Build history of the part. All positions in model axes, mm. A direction names the side the tool comes from. Coordinates: 2 decimals unless noted, no trailing zeros. Loops run counter-clockwise (first coordinate to the right, second up) from the corner with the lowest first, then second, coordinate; pieces in that order, holes last.
Item 1: Mould opens along X. For faces 3 (the face through (21, 2.54, -19)), 4 (the face through (0, 6.35, -19)), 5 (the face through (19.32, 1.25, -6.26)) say: released by +X, released by -X, zero draft, split by the parting line, or undercut.
Item 2: Cut at B-B (x = 25). List the corners of the cut face in (y, z), and give its area (3 significant figures).
Item 3: Flat gauge pins, fed straight in: pin 1 (2 mm diameter, centred on x = 20.5, y = 2.5, fed in from -Z); pin 2 (1.5 mm diameter, centred on y = 7.5, z = -30, fed in from +X); pin 3 (1 mm diameter, centred on y = 6.5, z = -32, fed in from -X). Where does each tip first touch, or does it go through?
Item 4: Cut at C-C (y = 4.75). List the corners of the cut face in (x, z) (3 decimals), and give its area (3 significant figures).
Item 5: Drill centre lines: line 1 along Y through (x, z) = (8, -12.5); line 2 along Y through (x, z) = (2, -21.5); line 3 along X through (y, z) = (4, -15.5). Where is each one in solid material? Low to high.
Item 6: 3-axis set-ups, long thin cutter, end or side, ignore diameter. For faces 1 (the face through (44.423, 5.671, -34.301)), 2 (the face through (-6.35, 1.25, -18.91)): which of +Z, -Z, +X, -X, +Y, -Y reach the whole face in a straight line?
Item 7: Cut at D-D (y = 8). List the corners of the cut face in (x, z), and give its area (3 significant figures).
Item 8: Cut at A-A (z = -19.05). List the corners of the cut face in (x, y) (3 decimals), and give its area (3 significant figures).
from build123d import *

# Parameters (mm, degrees)
BOSS_EXTRUDE1_DEPTH = 2.54
SKETCH2_R           = 16.51
BOSS_EXTRUDE2_DEPTH = 6.35
SKETCH3_R           = 4.445
BOSS_EXTRUDE3_DEPTH = 3.81


with BuildPart() as part:
    # Sketch1 → Boss-Extrude1 (new body)
    with BuildSketch(Plane(origin=(0, 0, 0), x_dir=(1, 0, 0), z_dir=(0, 1, 0))):
        with BuildLine():
            Line((0, 25.4), (38.1, 38.1))
            ThreePointArc((38.1, 38.1), (57.15, 19.05), (38.1, 0))
            Line((38.1, 0), (0, 12.7))
            ThreePointArc((0, 12.7), (-6.35, 19.05), (0, 25.4))
        make_face()
    extrude(amount=BOSS_EXTRUDE1_DEPTH)

    # Sketch2 → Boss-Extrude2 (add)
    with BuildSketch(Plane(origin=(0, 2.54, 0), x_dir=(1, 0, 0), z_dir=(0, 1, 0))):
        with Locations(Location((38.1, 19.05, 0), (0, 0, 90))):
            Circle(SKETCH2_R)
    extrude(amount=BOSS_EXTRUDE2_DEPTH)

    # Sketch3 → Boss-Extrude3 (add)
    with BuildSketch(Plane(origin=(0, 2.54, 0), x_dir=(1, 0, 0), z_dir=(0, 1, 0))):
        with Locations(Location((0, 19.05, 0), (0, 0, 90))):
            Circle(SKETCH3_R)
    extrude(amount=BOSS_EXTRUDE3_DEPTH)


solid = part.part
Filled sheet:
1. face 3: undercut
1. face 4: zero draft
1. face 5: released by -X
2. outline: (0, -33.73) - (2.54, -33.73) - (2.54, -29.1) - (8.89, -29.1) - (8.89, -9) - (2.54, -9) - (2.54, -4.37) - (0, -4.37) - close
2. area: 202 mm2
3. pin 1: stops at z = -32.57
3. pin 2: stops at x = 51.08
3. pin 3: stops at x = 27.26
4. outline: circle Ø8.89 at (0, -19.05); circle Ø33.02 at (38.1, -19.05)
4. area: 918 mm2
5. line 1: y = 0 to 2.54
5. line 2: y = 0 to 6.35
5. line 3: x = -2.67 to 2.67, 21.98 to 54.22
6. face 1: +Y
6. face 2: -X, +Y, -Y
7. outline: circle Ø33.02 at (38.1, -19.05)
7. area: 856 mm2
8. outline: (-6.35, 0) - (57.15, 0) - (57.15, 2.54) - (54.61, 2.54) - (54.61, 8.89) - (21.59, 8.89) - (21.59, 2.54) - (4.445, 2.54) - (4.445, 6.35) - (-4.445, 6.35) - (-4.445, 2.54) - (-6.35, 2.54) - close
8. area: 405 mm2
